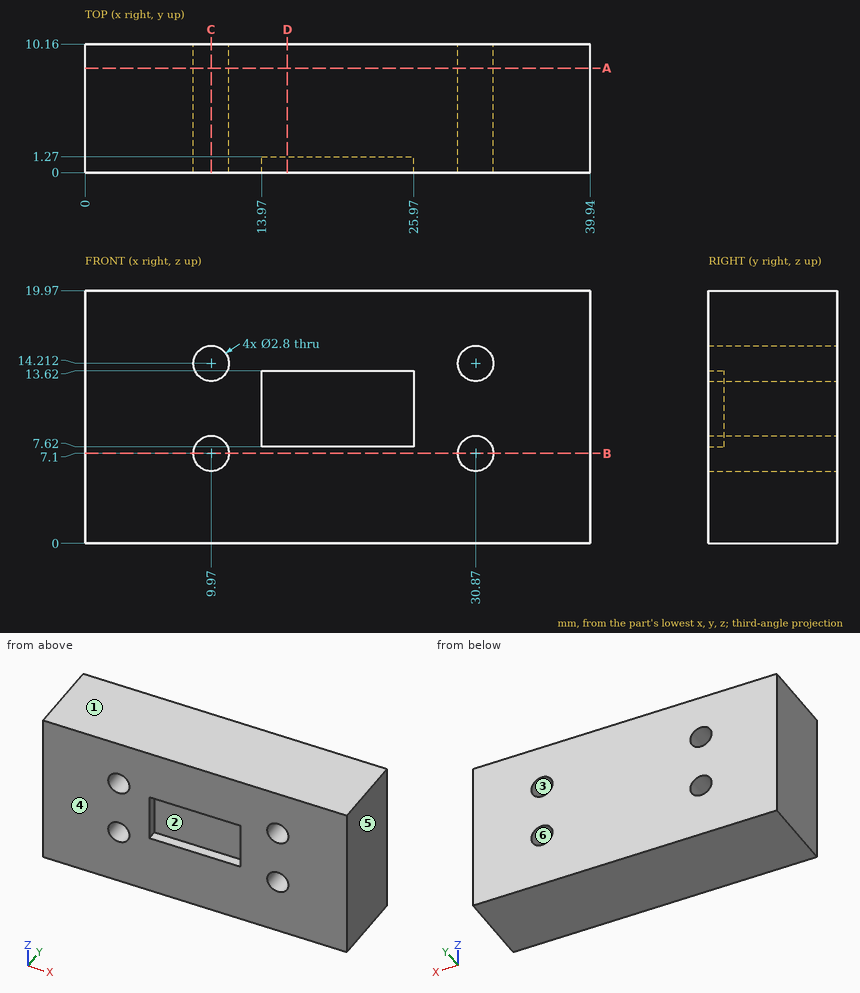
The figure shows three views and two pictorial views of one solid part (mm, origin at its lowest corner). Answer the questions. A direction names the side the tool comes from. Round coordinates to 2 decimals unless told otherwise and drop trailing zeros. Order: outer loops, then holes, each group sorted by start corner. A loop starts at its lowest first (then second) coordinate and runs counter-clockwise, first axis right, second up. Notation, with made-up numbers: (35.5, 7) - (83.5, 7) arc R17 ccw to (83.5, 27) - close; hole circle Ø3 at (-25, 3). An arc over 180 degrees is marked (long way). Write item = value, one per line. Start each with the question number.
1) Section B-B, the plane z = 7.1 is taken. Write down the section's boundary in (x, y), plus the area to 3 significant figures.
2) Section C-C, the plane x = 9.97 is taken. Write down the section's boundary in (y, z), plus the area to 3 significant figures.
3) For the marked faces 1 and 2, determine the directions among +Z, -Z, +X, -X, +Y, -Y from which every point of the face is accessible in a straight line to the end or side of a thin tool.
4) For a pull along X with two mould halves and no side action, classify the marked faces 3, 4, 5 and 6 as released by +X, released by -X, zero draft, split by the parting line, or undercut.
5) Section D-D, the plane x = 16 is taken. Write down the section's boundary in (y, z).
6) Straight lines are drawn through the part: L1, parallel to X at y = 6.75, z = 7; L2, parallel to X at y = 2.75, z = 8.25. For each, find the intervals that lie inside material, in ascending order.
7) Given pin 1 (1 mm diameter, centred on x = 21, y = 0.5, fed in from -Z), flat-ended and moving along its own axis, determine where the tip first touches the part or whether it passes through.
8) Section A-A, the plane y = 8.25 is taken. Write down the section's boundary in (x, z), plus the area to 3 significant figures.
Results list:
q1.outline = (0, 0) - (8.57, 0) - (8.57, 10.16) - (0, 10.16) - close; (11.37, 0) - (29.47, 0) - (29.47, 10.16) - (11.37, 10.16) - close; (32.27, 0) - (39.94, 0) - (39.94, 10.16) - (32.27, 10.16) - close
q1.area = 349 mm^2
q2.outline = (0, 0) - (10.16, 0) - (10.16, 5.7) - (0, 5.7) - close; (0, 8.5) - (10.16, 8.5) - (10.16, 12.81) - (0, 12.81) - close; (0, 15.61) - (10.16, 15.61) - (10.16, 19.97) - (0, 19.97) - close
q2.area = 146 mm^2
q3.face_1 = +Z, +X, -X, +Y, -Y
q3.face_2 = -Y
q4.face_3 = undercut
q4.face_4 = zero draft
q4.face_5 = released by +X
q4.face_6 = undercut
q5.outline = (0, 0) - (10.16, 0) - (10.16, 19.97) - (0, 19.97) - (0, 13.62) - (1.27, 13.62) - (1.27, 7.62) - (0, 7.62) - close
q6.L1 = 0 to 8.57, 11.37 to 29.47, 32.27 to 39.94
q6.L2 = 0 to 9.17, 10.77 to 30.07, 31.67 to 39.94
q7.pin_1 = 0
q8.outline = (0, 0) - (39.94, 0) - (39.94, 19.97) - (0, 19.97) - close; hole circle Ø2.8 at (9.97, 7.1); hole circle Ø2.8 at (9.97, 14.21); hole circle Ø2.8 at (30.87, 7.1); hole circle Ø2.8 at (30.87, 14.21)
q8.area = 773 mm^2
